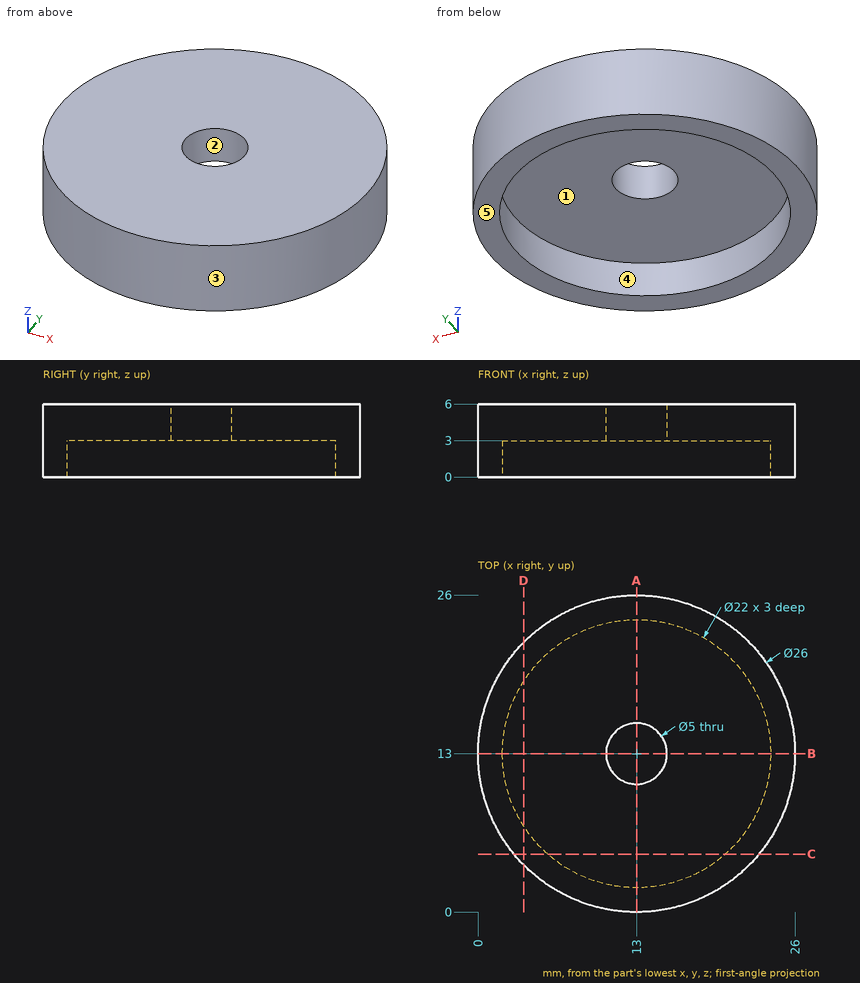
Design review of the part shown in the three views and the two pictorial views. Dimensions are in mm from the part's minimum x, y and z. A direction names the side the tool comes from. Round coordinates to 2 decimals unless told otherwise and drop trailing zeros. Loops run counter-clockwise (first coordinate to the right, second up) from the corner with the lowest first, then second, coordinate; pieces in that order, holes last. Notation, with made-up numbers: (34, 34) - (40, 34) arc R13 cw to (40, 47) - close; hole circle Ø3 at (15.5, 9.5). An arc over 180 degrees is marked (long way). One line per item, written item: value. Start each with the question number.
Item 1: Take a section at C-C (y = 4.75). Give the boundary of the cut face in (x, z), plus the area to 3 significant figures.
Item 2: For the marked faces 1 and 2, list the 3-axis set-ups (+Z, -Z, +X, -X, +Y, -Y) from which the entire face can be reached by the end or side of a thin tool; tool diameter is ignored.
Item 3: For L1, parallel to Y at x = 13, z = 3.85; L2, parallel to Y at x = 13, z = 0.9; L3, parallel to Z at x = 15, y = 7.5, list the stretches that pass through material, from the lowest coordinate up.
Item 4: The part is to be moulded in two halves that separate along X. For the marked faces 3, 4 and 5, say which applies: +X half, -X half, draft (parallel to the pull), parting line (faces both ways), or undercut.
Item 5: Take a section at D-D (x = 3.75). Give the boundary of the cut face in (y, z).
Item 6: Take a section at A-A (x = 13). Give the boundary of the cut face in (y, z).
Item 7: Clearance check with flat-ended pins moving along their axes: pin 1 Ø2 at (x, z) = (21, 1) entering from +Y; pin 2 Ø8 at (x, y) = (13, 13) entering from -Z; pin 3 Ø3 at (x, z) = (20.5, 2.5) entering from +Y. State where each tip first meets the part, or that it passes through.
Answer below:
1. outline: (2.95, 0) - (5.72, 0) - (5.72, 3) - (20.28, 3) - (20.28, 0) - (23.05, 0) - (23.05, 6) - (2.95, 6) - close
1. area: 76.9 mm2
2. face 1: -Z
2. face 2: +Z, -Z
3. L1: y = 0 to 10.5, 15.5 to 26
3. L2: y = 0 to 2, 24 to 26
3. L3: z = 3 to 6
4. face 3: parting line
4. face 4: undercut
4. face 5: draft
5. outline: (3.87, 0) - (7.05, 0) - (7.05, 3) - (18.95, 3) - (18.95, 0) - (22.13, 0) - (22.13, 6) - (3.87, 6) - close
6. outline: (0, 0) - (2, 0) - (2, 3) - (10.5, 3) - (10.5, 6) - (0, 6) - close; (15.5, 3) - (24, 3) - (24, 0) - (26, 0) - (26, 6) - (15.5, 6) - close
7. pin 1: stops at y = 23.95
7. pin 2: stops at z = 3
7. pin 3: stops at y = 24.53
